Part print with two shaded views. Sizes in mm from the minimum x, y, z corner. Coordinates: 2 decimals unless noted, no trailing zeros. Loops run counter-clockwise (first coordinate to the right, second up) from the corner with the lowest first, then second, coordinate; pieces in that order, holes last.
(1) Slice it at B-B (x = 16). Give the cut face in (y, z).
(2) Slice it at A-A (z = 0.4). Give the cut face in (x, y), and give its area (3 significant figures).
(3) Two-plate mould, pull along X, no slides. Class the marked faces 1, 2 and 3: pulls with the +X half, pulls with the -X half, needs draft (parallel to the pull), parting line crosses it, or undercut.
(4) Slice it at D-D (z = 2.4). Give the cut face in (x, y).
(5) Wall check: L1, parallel to X at y = 2.5, z = 1.3; L2, parallel to X at y = 7.25, z = 2.6; L3, parallel to X at y = 7.75, z = 0.85. Give the ranges that are in metal, low to high.
(6) Slice it at C-C (y = 9.25). Give the cut face in (x, z), and give its area (3 significant figures).
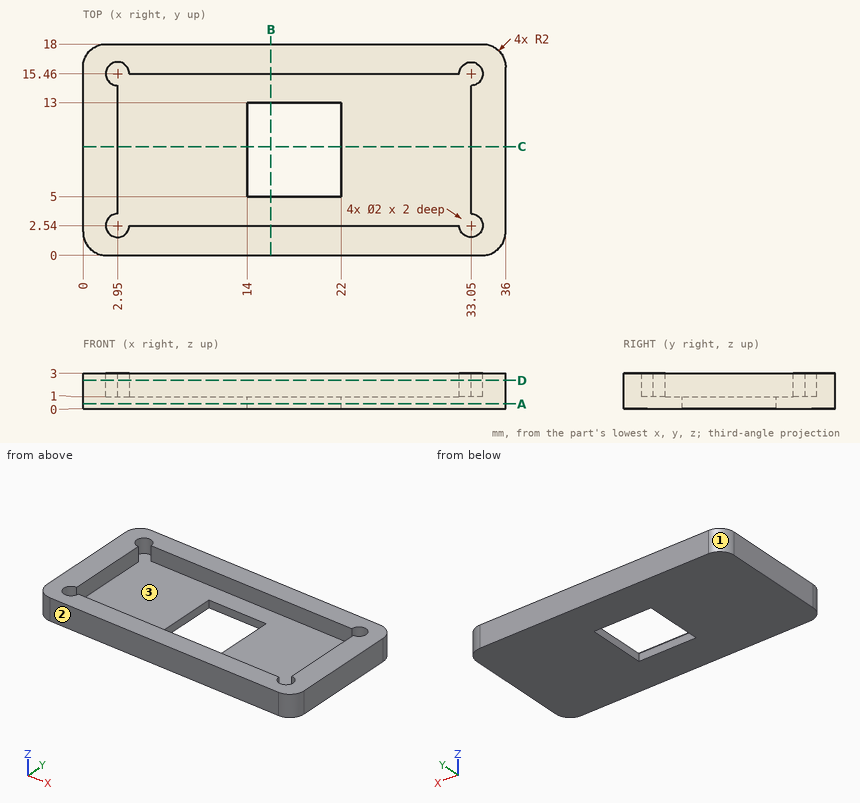
Response values:
1. outline: (0, 0) - (5, 0) - (5, 1) - (2.54, 1) - (2.54, 3) - (0, 3) - close; (13, 0) - (18, 0) - (18, 3) - (15.46, 3) - (15.46, 1) - (13, 1) - close
2. outline: (0, 2) arc R2 ccw to (2, 0) - (34, 0) arc R2 ccw to (36, 2) - (36, 16) arc R2 ccw to (34, 18) - (2, 18) arc R2 ccw to (0, 16) - close; hole (14, 5) - (22, 5) - (22, 13) - (14, 13) - close
2. area: 581 mm2
3. face 1: pulls with the -X half
3. face 2: needs draft
3. face 3: undercut
4. outline: (0, 2) arc R2 ccw to (2, 0) - (34, 0) arc R2 ccw to (36, 2) - (36, 16) arc R2 ccw to (34, 18) - (2, 18) arc R2 ccw to (0, 16) - close; hole (2.95, 3.54) arc R1 ccw (long way) to (3.95, 2.54) - (32.05, 2.54) arc R1 ccw (long way) to (33.05, 3.54) - (33.05, 14.46) arc R1 ccw (long way) to (32.05, 15.46) - (3.95, 15.46) arc R1 ccw (long way) to (2.95, 14.46) - close
5. L1: x = 0 to 1.95, 3.95 to 32.05, 34.05 to 36
5. L2: x = 0 to 2.95, 33.05 to 36
5. L3: x = 0 to 14, 22 to 36
6. outline: (0, 0) - (14, 0) - (14, 1) - (2.95, 1) - (2.95, 3) - (0, 3) - close; (22, 0) - (36, 0) - (36, 3) - (33.05, 3) - (33.05, 1) - (22, 1) - close
6. area: 39.8 mm2
